from build123d import *

# Parameters (mm, degrees)
FILLET2_R  = 1.8
SKETCH2_W  = 12
SKETCH2_H  = 1.6
SLOT_DEPTH = 1.4


with BuildPart() as part:
    # BodySke → Base-Revolve (revolve)
    with BuildSketch(Plane.XY):
        Polygon((3.6, 3), (3.6, 6), (0, 5.685040811), (0, 0), (43.6, 0), (43.6, 3), align=None)
    revolve(axis=Axis((-25.4, 0, 0), (1, 0, 0)))

    # Fillet2
    fillet2_edges = [part.edges().sort_by_distance(p)[0] for p in [
        (0, -5.685040811, 0),
    ]]
    fillet(fillet2_edges, radius=FILLET2_R)

    # Sketch2 → Slot (cut)
    with BuildSketch(Plane(origin=(0, 0, 0), x_dir=(0, 0, -1), z_dir=(1, 0, 0))):
        Rectangle(SKETCH2_W, SKETCH2_H)
    extrude(amount=SLOT_DEPTH, mode=Mode.SUBTRACT)


solid = part.part
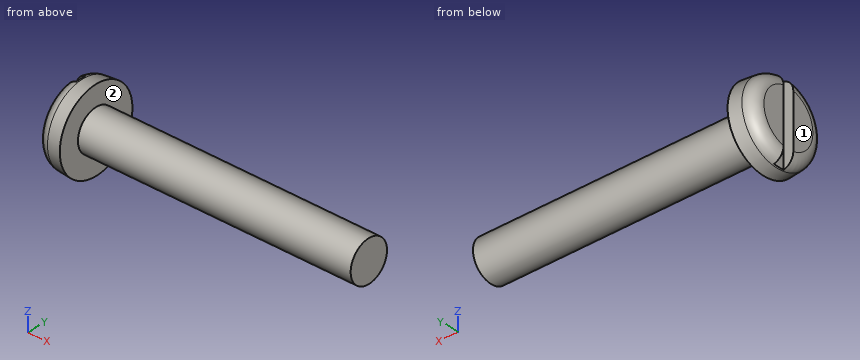
Source: CAD feature listing. Evaluate the final solid. Frame: model axes, mm. Face numbers are marked on the shaded views. A direction names the side the tool comes from. Give positions to 0.01 mm unless a question says otherwise; leave off trailing zeros. Write each loop counter-clockwise with the first axis right and the second up, starting at its lowest first coordinate (ties: lowest second). Pieces come first, ordered by that corner, then holes. Notation, with made-up numbers: M 81,81.25 L 118,81.25 A16 cw 118,97.25 Z; hole C 70,71.25 d6. An arc over 180 degrees is marked long. Return JSON: item names as keys, results as strings. Group by question number.
1) Set-up query: the marked faces 1 and 2. Return all of +Z, -Z, +X, -X, +Y, -Y with unobstructed straight access to the full face (end or side cutting, diameter ignored); none if empty.
2) Cut plane C-C, the plane x = 23.5. Output: boundary loops of the cut face in (y, z).
3) Cut plane B-B, the plane y = 0. Output: boundary loops of the cut face in (x, z), then the cut area to 3 significant figures.
4) Ray query, L1, parallel to X at y = -0.5, z = 1; L2, parallel to X at y = -2.5, z = 2.75; L3, parallel to Z at x = 22.5, y = 0. Return the intervals inside material, ascending.
5) First-contact query: pin 1 Ø5 at (x, y) = (31.5, -1.5) entering from -Z; pin 2 Ø5 at (y, z) = (4.5, 4) entering from +X; pin 3 Ø1 at (x, z) = (38.5, 0) entering from -Y; pin 4 Ø1 at (y, z) = (1, -3) entering from -X. Flat tips, straight axial feed; report the tip coordinate or a pass-through.
6) Cut plane A-A, the plane z = 0. Output: boundary loops of the cut face in (x, y), then the cut area to 3 significant figures.
Data:
{
 "1": {"face 1": "+Z, -Z, -X, +Y, -Y", "face 2": "+X"},
 "2": {"outline": "C 0,0 d6"},
 "3": {"outline": "M 1.4,-5.79 A1.8 ccw 1.64,-5.83 L 3.6,-6 L 3.6,-3 L 43.6,-3 L 43.6,3 L 3.6,3 L 3.6,6 L 1.64,5.83 A1.8 ccw 1.4,5.79 Z", "area": "266 mm²"},
 "4": {"L1": "x = 1.4 to 43.6", "L2": "x = 0 to 3.6", "L3": "z = -3 to 3"},
 "5": {"pin 1": "stops at z = -3", "pin 2": "stops at x = 3.6", "pin 3": "stops at y = -3", "pin 4": "stops at x = 0"},
 "6": {"outline": "M 0,-4.04 A1.8 ccw 1.64,-5.83 L 3.6,-6 L 3.6,-3 L 43.6,-3 L 43.6,3 L 3.6,3 L 3.6,6 L 1.64,5.83 A1.8 ccw 0,4.04 L 0,0.8 L 1.4,0.8 L 1.4,-0.8 L 0,-0.8 Z", "area": "279 mm²"}
}
